from build123d import *

# Parameters (mm, degrees)
SKETCH1_R                  = 22.225
SKETCH1_R_2                = 14.2875
SKETCH1_R_3                = 12.065
BOSS_EXTRUDE1_DEPTH        = 6.35
F_9_0_196_DIAMETER_HOLE1_D = 4.9784


with BuildPart() as part:
    # Sketch1 → Boss-Extrude1 (new body)
    with BuildSketch(Plane(origin=(0, 0, 0), x_dir=(0, 1, 0), z_dir=(0, 0, 1))):
        with BuildLine():
            Line((80.9625, -82.55), (80.9625, -139.7))
            Line((80.9625, -139.7), (-165.481, -139.7))
            Line((-165.481, -139.7), (-165.481, -8.2804))
            Line((-165.481, -8.2804), (-27.237142114, 57.361904514))
            ThreePointArc((-27.237142114, 57.361904514), (28.32715108, 56.831527444), (62.200093141, 12.782738878))
            Line((62.200093141, 12.782738878), (80.150058213, -74.560788201))
            ThreePointArc((80.150058213, -74.560788201), (80.758867143, -78.534792445), (80.9625, -82.55))
        make_face()
        with Locations(Location((0, 0, 0), (0, 0, 270))):
            Circle(SKETCH1_R, mode=Mode.SUBTRACT)
        with Locations(Location((-41.275, -82.55, 0), (0, 0, 270))):
            Circle(SKETCH1_R_2, mode=Mode.SUBTRACT)
        with Locations(Location((41.275, -82.55, 0), (0, 0, 270))):
            Circle(SKETCH1_R_2, mode=Mode.SUBTRACT)
        with Locations(Location((-114.3, -41.275, 0), (0, 0, 270))):
            Circle(SKETCH1_R_3, mode=Mode.SUBTRACT)
    extrude(amount=BOSS_EXTRUDE1_DEPTH)

    # #9 (0.196) Diameter Hole1 (through all)
    with Locations(Plane.XY.offset(6.35)):
        with Locations((127, 75.819), (82.55, -41.275), (82.55, 41.275), (57.15, 41.275), (82.55, 66.675), (107.95, 41.275), (82.55, 15.875), (82.55, -15.875), (57.15, -41.275), (82.55, -66.675), (107.95, -41.275), (127, -152.781), (127, -140.081), (127, -127.381), (127, -114.681), (127, -101.981), (127, -89.281), (127, -76.581), (127, -63.881), (127, -51.181), (127, -38.481), (127, -25.781), (127, -13.081), (-17.927602772, -71.974049098), (-10.756561663, -79.171393707), (0, -89.96741062), (41.275, -112.8014), (74.2696, -114.3), (41.275, -152.781), (8.2804, -114.3), (127, -0.381), (127, 12.319), (127, 25.019), (127, 37.719), (127, 50.419), (127, 63.119)):
            Hole(F_9_0_196_DIAMETER_HOLE1_D / 2)


solid = part.part
Verification items for the finished model (mm, model axes). Give positions to 0.01 mm unless a question says otherwise; leave off trailing zeros.
1) Sectioned sample at A-A, the plane z = 5. Count the separate pieces of the cut face and the enclosed holes in it, then the cut area to 3 significant figures.
2) Thickness scan on line 1 along Y through (x, z) = (0, 4.5) (3 decimals); line 2 along X through (y, z) = (39, 1.5); line 3 along Y through (x, z) = (-17, 4.5). Record the ranges inside material, lowest first.
3) Draft check along X on faces 1 (the flat face through (139.7, -41, 3)), 2 (the flat face through (111, 80.962, 3)), 3 (the cylindrical face through (124.626, -139.333, 3.131)). Enter one of: pulls with the +X half, pulls with the -X half, needs draft (parallel to the pull), parting line crosses it, or undercut.
4) Depth check by flat-ended pin: pin 1 Ø8 at (x, y) = (41.275, -152.781) entering from -Z; pin 2 Ø1.5 at (y, z) = (-63.5, 2) entering from -X. Enter the tip coordinate at first touch or a pass-through.
Answers:
1. separate pieces: 1
1. enclosed holes: 37
1. area: 38,100 mm2
2. line 1: y = -148.042 to -92.457, -87.478 to -22.225, 22.225 to 64.827
2. line 2: x = -50.11 to 56.14, 58.16 to 68.44, 96.66 to 106.94, 108.96 to 124.87, 129.13 to 139.7
2. line 3: y = -112.24 to -74.28, -69.66 to -14.32, 14.32 to 61.18
3. face 1: pulls with the +X half
3. face 2: needs draft
3. face 3: undercut
4. pin 1: stops at z = 0
4. pin 2: stops at x = -40.5
